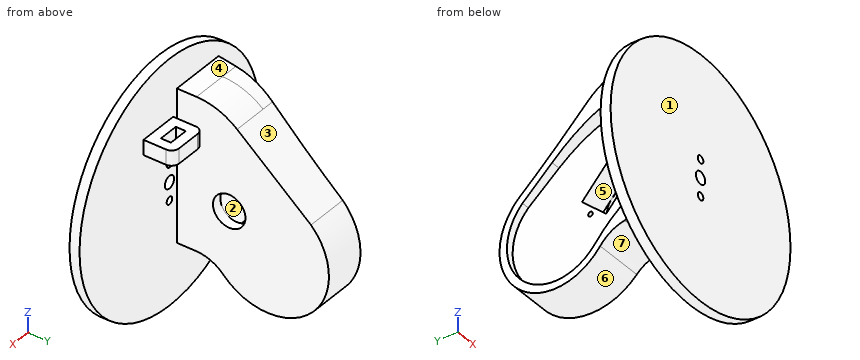
```python
from build123d import *

# Parameters (mm, degrees)
SKETCH2_R                       = 48.5
BOSS_EXTRUDE1_DEPTH             = 4
SKETCH4_R                       = 1.5
CUT_EXTRUDE2_DEPTH              = 69.705894944
SKETCH5_R                       = 2.5
CUT_EXTRUDE3_DEPTH              = 69.705894944
BOSS_EXTRUDE2_DEPTH             = 14
BOSS_EXTRUDE7_DEPTH             = 9
BOSS_EXTRUDE7_DIRECTION_2_REACH = 104.912
BOSS_EXTRUDE10_DEPTH            = 9
SKETCH27_W                      = 16
SKETCH27_H                      = 6
BOSS_EXTRUDE11_DEPTH            = 12
FILLET6_R                       = 3
CUT_EXTRUDE16_REACH             = 111.016
SKETCH28_W                      = 8
SKETCH28_H                      = 4
CUT_EXTRUDE17_DEPTH             = 95.342420983
CUT_EXTRUDE17_DEPTH_BACK        = 95.342420983
SKETCH31_R                      = 6.5
CUT_EXTRUDE18_DEPTH             = 105.740118374
CUT_EXTRUDE19_DEPTH             = 10
SKETCH32_R                      = 0.92049896
CUT_EXTRUDE20_DEPTH             = 4
SKETCH32_3_R                    = 0.92049896
CUT_EXTRUDE21_DEPTH             = 4


with BuildPart() as part:
    # Sketch2 → Boss-Extrude1 (new body)
    with BuildSketch(Plane(origin=(0, 0, 0), x_dir=(1, 0, 0), z_dir=(0, 1, 0))):
        with Locations(Location((0, 0, 0), (0, 0, 270))):
            Circle(SKETCH2_R)
    extrude(amount=BOSS_EXTRUDE1_DEPTH)

    # Sketch4 → Cut-Extrude2 (cut, through all)
    with BuildSketch(Plane.XZ):
        with Locations(Location((0, 7.25, 0), (0, 0, 270))):
            Circle(SKETCH4_R)
        with Locations(Location((0, -7.25, 0), (0, 0, 270))):
            Circle(SKETCH4_R)
    extrude(amount=-CUT_EXTRUDE2_DEPTH, mode=Mode.SUBTRACT)

    # Sketch5 → Cut-Extrude3 (cut, through all)
    with BuildSketch(Plane.XZ):
        with Locations(Location((0, 0, 0), (0, 0, 270))):
            Circle(SKETCH5_R)
    extrude(amount=-CUT_EXTRUDE3_DEPTH, mode=Mode.SUBTRACT)

    # Sketch7 → Boss-Extrude2 (add)
    with BuildSketch(Plane(origin=(-4, 0, 0), x_dir=(0, 0, -1), z_dir=(1, 0, 0))):
        with BuildLine():
            Line((23.129947874, 4), (23.129947874, 11.644549616))
            ThreePointArc((23.129947874, 11.644549616), (24.589048403, 18.743749901), (28.729797284, 24.692011643))
            ThreePointArc((28.729797284, 24.692011643), (29.313383054, 55.284736897), (-1.284289494, 55.479275971))
            Line((-1.284289494, 55.479275971), (-27.227315747, 29.536249718))
            ThreePointArc((-27.227315747, 29.536249718), (-32.64663453, 21.425665997), (-34.549646217, 11.858580188))
            Line((-34.549646217, 11.858580188), (-34.549646217, 4))
            Line((-34.549646217, 4), (23.129947874, 4))
        make_face()
    extrude(amount=-BOSS_EXTRUDE2_DEPTH)

    # Sketch17 → Boss-Extrude7 (add)
    with BuildSketch(Plane.ZY.offset(18)):
        with BuildLine():
            ThreePointArc((34.549646217, 11.858580188), (33.008342843, 20.500891953), (28.574482006, 28.077569775))
            ThreePointArc((28.574482006, 28.077569775), (27.915386359, 28.820289685), (27.227315747, 29.536249718))
            Line((27.227315747, 29.536249718), (1.284289494, 55.479275971))
            Line((1.284289494, 55.479275971), (26.295003593, 26.127182305))
            ThreePointArc((26.295003593, 26.127182305), (30.194232218, 19.461281607), (31.549646217, 11.858580188))
            Line((31.549646217, 11.858580188), (31.549646217, 4))
            Line((31.549646217, 4), (34.549646217, 4))
            Line((34.549646217, 4), (34.549646217, 11.858580188))
        make_face()
        with BuildLine():
            Line((28.574482006, 28.077569775), (3.405609837, 57.600596315))
            ThreePointArc((3.405609837, 57.600596315), (-31.461505391, 57.378912253), (-30.796489049, 22.517434639))
            ThreePointArc((-30.796489049, 22.517434639), (-27.345864981, 17.560549854), (-26.129947874, 11.644549616))
            Line((-26.129947874, 11.644549616), (-26.129947874, 4))
            Line((-26.129947874, 4), (-23.129947874, 4))
            Line((-23.129947874, 4), (-23.129947874, 11.644549616))
            ThreePointArc((-23.129947874, 11.644549616), (-24.589048403, 18.743749901), (-28.729797284, 24.692011643))
            ThreePointArc((-28.729797284, 24.692011643), (-29.313383054, 55.284736897), (1.284289494, 55.479275971))
            Line((1.284289494, 55.479275971), (27.227315747, 29.536249718))
            ThreePointArc((27.227315747, 29.536249718), (27.915386359, 28.820289685), (28.574482006, 28.077569775))
        make_face()
    extrude(amount=BOSS_EXTRUDE7_DEPTH)

    # Boss-Extrude7 direction 2: up to this face of the body (flat: up to its plane)
    boss_extrude7_direction_2_end = Plane(part.part.faces().sort_by_distance((-4, 29.339157607, -2.736239069))[0])
    # Sketch17 → Boss-Extrude7 direction 2 (add, up to the picked face)
    with BuildSketch(Plane.ZY.offset(18), mode=Mode.PRIVATE) as boss_extrude7_direction_2_sk1:
        with BuildLine():
            ThreePointArc((34.549646217, 11.858580188), (33.008342843, 20.500891953), (28.574482006, 28.077569775))
            ThreePointArc((28.574482006, 28.077569775), (27.915386359, 28.820289685), (27.227315747, 29.536249718))
            Line((27.227315747, 29.536249718), (1.284289494, 55.479275971))
            Line((1.284289494, 55.479275971), (26.295003593, 26.127182305))
            ThreePointArc((26.295003593, 26.127182305), (30.194232218, 19.461281607), (31.549646217, 11.858580188))
            Line((31.549646217, 11.858580188), (31.549646217, 4))
            Line((31.549646217, 4), (34.549646217, 4))
            Line((34.549646217, 4), (34.549646217, 11.858580188))
        make_face()
    boss_extrude7_direction_2_tool1 = split(extrude(boss_extrude7_direction_2_sk1.sketch, amount=-BOSS_EXTRUDE7_DIRECTION_2_REACH, mode=Mode.PRIVATE), bisect_by=boss_extrude7_direction_2_end, keep=Keep.BOTH, mode=Mode.PRIVATE)
    # Sketch17 → Boss-Extrude7 direction 2 (add, up to the picked face)
    with BuildSketch(Plane.ZY.offset(18), mode=Mode.PRIVATE) as boss_extrude7_direction_2_sk2:
        with BuildLine():
            Line((28.574482006, 28.077569775), (3.405609837, 57.600596315))
            ThreePointArc((3.405609837, 57.600596315), (-31.461505391, 57.378912253), (-30.796489049, 22.517434639))
            ThreePointArc((-30.796489049, 22.517434639), (-27.345864981, 17.560549854), (-26.129947874, 11.644549616))
            Line((-26.129947874, 11.644549616), (-26.129947874, 4))
            Line((-26.129947874, 4), (-23.129947874, 4))
            Line((-23.129947874, 4), (-23.129947874, 11.644549616))
            ThreePointArc((-23.129947874, 11.644549616), (-24.589048403, 18.743749901), (-28.729797284, 24.692011643))
            ThreePointArc((-28.729797284, 24.692011643), (-29.313383054, 55.284736897), (1.284289494, 55.479275971))
            Line((1.284289494, 55.479275971), (27.227315747, 29.536249718))
            ThreePointArc((27.227315747, 29.536249718), (27.915386359, 28.820289685), (28.574482006, 28.077569775))
        make_face()
    boss_extrude7_direction_2_tool2 = split(extrude(boss_extrude7_direction_2_sk2.sketch, amount=-BOSS_EXTRUDE7_DIRECTION_2_REACH, mode=Mode.PRIVATE), bisect_by=boss_extrude7_direction_2_end, keep=Keep.BOTH, mode=Mode.PRIVATE)
    add(boss_extrude7_direction_2_tool1.solids().sort_by(Axis((-18, 4.612919, 33.049646), (1, 0, 0)))[0])
    add(boss_extrude7_direction_2_tool2.solids().sort_by(Axis((-18, 43.147366, 14.895406), (1, 0, 0)))[0])

    # Sketch25 → Boss-Extrude10 (add)
    with BuildSketch(Plane.ZY.offset(18)):
        with BuildLine():
            ThreePointArc((-28.729797284, 24.692011643), (-24.589048403, 18.743749901), (-23.129947874, 11.644549616))
            Line((-23.129947874, 11.644549616), (-23.129947874, 4))
            Line((-23.129947874, 4), (-15.129947874, 4))
            add(Edge.make_bspline(
                [(-28.729797284, 24.692011643), (-21.954867515, 18.253200081), (-19.09405247, 12.798017691), (-15.129947874, 4)],
                knots=[0, 0, 0, 0, 1, 1, 1, 1], degree=3))
        make_face()
        with BuildLine():
            add(Edge.make_bspline(
                [(11.751619577, 43.19501844), (26.551255916, 25.8264495), (25.549646217, 4)],
                knots=[0, 0, 0, 1, 1, 1], degree=2))
            Line((25.549646217, 4), (31.549646217, 4))
            Line((31.549646217, 4), (31.549646217, 11.858580188))
            ThreePointArc((31.549646217, 11.858580188), (30.194232218, 19.461281607), (26.295003593, 26.127182305))
            Line((26.295003593, 26.127182305), (11.751619577, 43.19501844))
        make_face()
    extrude(amount=BOSS_EXTRUDE10_DEPTH)

    # Sketch27 → Boss-Extrude11 (add)
    with BuildSketch(Plane(origin=(0, 4, 0), x_dir=(1, 0, 0), z_dir=(0, 1, 0))):
        with Locations((6, -21.549646217)):
            Rectangle(SKETCH27_W, SKETCH27_H)
    extrude(amount=BOSS_EXTRUDE11_DEPTH)

    # Fillet6
    fillet6_edges = [part.edges().sort_by_distance(p)[0] for p in [
        (-2, 16, 21.549646217),
        (14, 16, 21.549646217),
    ]]
    fillet(fillet6_edges, radius=FILLET6_R)

    # Sketch28 → Cut-Extrude16 (cut, up to next)
    with BuildSketch(Plane.XY.offset(24.549646217), mode=Mode.PRIVATE) as cut_extrude16_sk1:
        with Locations((6, 10)):
            Rectangle(SKETCH28_W, SKETCH28_H)
    cut_extrude16_tool1 = extrude(cut_extrude16_sk1.sketch, amount=-CUT_EXTRUDE16_REACH, mode=Mode.PRIVATE) & part.part
    add(cut_extrude16_tool1.solids().sort_by_distance((6, 10, 24.549646))[0], mode=Mode.SUBTRACT)

    # Sketch29 → Cut-Extrude17 (cut, two sides: drawn at the far end of the back side and taken through both)
    with BuildSketch(Plane.XY.offset(-CUT_EXTRUDE17_DEPTH_BACK)):
        with BuildLine():
            Line((-21, 64.776480176), (-27, 64.776480176))
            Line((-27, 64.776480176), (-27, 4))
            Line((-27, 4), (-26.5, 4))
            add(Edge.make_bspline(
                [(-21, 64.776480176), (-21.220459696, 34.140901434), (-26.5, 4)],
                knots=[0, 0, 0, 1, 1, 1], degree=2))
        make_face()
    extrude(amount=CUT_EXTRUDE17_DEPTH + CUT_EXTRUDE17_DEPTH_BACK, mode=Mode.SUBTRACT)

    # Sketch31 → Cut-Extrude18 (cut, through all)
    with BuildSketch(Plane.ZY.offset(18)):
        with Locations((-4.922469695, 24.905412087)):
            Circle(SKETCH31_R)
    extrude(amount=-CUT_EXTRUDE18_DEPTH, mode=Mode.SUBTRACT)

    # Sketch31<3> → Cut-Extrude19 (cut)
    with BuildSketch(Plane.ZY.offset(18)):
        Polygon((-5.41546104, 34.054639751), (11.74960782, 18.74580534), (3.09678837, 9.043809897), (-14.06828049, 24.352644308), align=None)
    extrude(amount=-CUT_EXTRUDE19_DEPTH, mode=Mode.SUBTRACT)

    # Sketch32 → Cut-Extrude20 (cut)
    with BuildSketch(Plane.ZY.offset(18)):
        with Locations((-11.584503567, 30.654960303)):
            Circle(SKETCH32_R)
    extrude(amount=-CUT_EXTRUDE20_DEPTH, mode=Mode.SUBTRACT)

    # Sketch32<3> → Cut-Extrude21 (cut)
    with BuildSketch(Plane.ZY.offset(18)):
        with Locations((-11.584503567, 30.654960303)):
            Circle(SKETCH32_3_R)
        with Locations(Location((10.118376889, 12.711132154, 0), (0, 0, 180))):
            Circle(SKETCH32_3_R)
    extrude(amount=-CUT_EXTRUDE21_DEPTH, mode=Mode.SUBTRACT)


solid = part.part
```
Source: CAD feature listing. Evaluate the final solid. Frame: model axes, mm. Face numbers are marked on the shaded views. A direction names the side the tool comes from. Round coordinates to 2 decimals unless told otherwise and drop trailing zeros. Loops run counter-clockwise (first coordinate to the right, second up) from the corner with the lowest first, then second, coordinate; pieces in that order, holes last. Notation, with made-up numbers: (72, 28) - (112, 28) arc R27 cw to (112, 51) - close; hole circle Ø4 at (57.5, 75.5). An arc over 180 degrees is marked (long way). Use CSV: the item, a comma, the result in double quotes.
Q1. Section query D-D, the plane z = -41.5. Output: boundary loops of the cut face in (x, y).
Reported:
outline,"(-25.1, 0) - (25.1, 0) - (25.1, 4) - (-25.1, 4) - close"
Q2. Reachability of the marked faces 5, 6 and 7 from +Z, -Z, +X, -X, +Y, -Y: full face, straight path, thin tool, end or side. Return the list, or none.
Reported:
face 5,"-X"
face 6,"+X, -X"
face 7,"-Z, +X, -X"
Q3. Section query B-B, the plane z = -7.25. Give the number of separate pieces and of enclosed holes in the cut face, then the cut area to 3 significant figures.
Reported:
separate pieces,"3"
enclosed holes,"0"
area,"1,030 mm^2"
Q4. Mould query, pull axis Y, two halves, no side actions, for the marked faces 1, 2, 3 and 4. Classes: pulls with the +Y half, pulls with the -Y half, needs draft (parallel to the pull), parting line crosses it, or undercut.
Reported:
face 1,"pulls with the -Y half"
face 2,"undercut"
face 3,"pulls with the +Y half"
face 4,"needs draft"
Q5. Pin query (flat end, axial travel): pin 1 Ø4 at (y, z) = (25.5, -11) entering from -X; pin 2 Ø5 at (x, z) = (5, 21) entering from +Y; pin 3 Ø6 at (x, z) = (-26.5, -9) entering from +Y; pin 4 Ø2.5 at (x, z) = (0, 7.25) entering from -Y (3 decimals). Return the tip coordinate at first contact, or that it passes through.
Reported:
pin 1,"x = -18"
pin 2,"y = 16"
pin 3,"y = 4"
pin 4,"through"
Q6. Section query A-A, the plane x = 8. Output: boundary loops of the cut face in (y, z), then the cut area to 3 significant figures.
Reported:
outline,"(0, -47.84) - (4, -47.84) - (4, 18.55) - (8, 18.55) - (8, 24.55) - (4, 24.55) - (4, 47.84) - (0, 47.84) - close; (12, 18.55) - (16, 18.55) - (16, 24.55) - (12, 24.55) - close"
area,"431 mm^2"
Q7. Section query C-C, the plane x = 22.5. Output: boundary loops of the cut face in (y, z), then the cut area to 3 significant figures.
Reported:
outline,"(0, -42.97) - (4, -42.97) - (4, 42.97) - (0, 42.97) - close"
area,"344 mm^2"
Q8. Ray query, line 1 along X through (y, z) = (2.25, 0); line 2 along Y through (x, z) = (-29.5, -7.5); line 3 along Y through (x, z) = (-10.5, 31). Return the intervals inside material, ascending.
Reported:
line 1,"-48.5 to -2.5, 2.5 to 48.5"
line 2,"0 to 4"
line 3,"0 to 24.7"
